Drawing for the job (mm, zero at the part's lowest x, y, z). Coordinates: 2 decimals unless noted, no trailing zeros. Loops run counter-clockwise (first coordinate to the right, second up) from the corner with the lowest first, then second, coordinate; pieces in that order, holes last. Notation, with made-up numbers: (-13, -24.75) - (27, -24.75) arc R3 ccw to (27, -20.75) - close; hole circle Ø11 at (-3.5, 2). An arc over 180 degrees is marked (long way). Put each result on its own line as item: value.
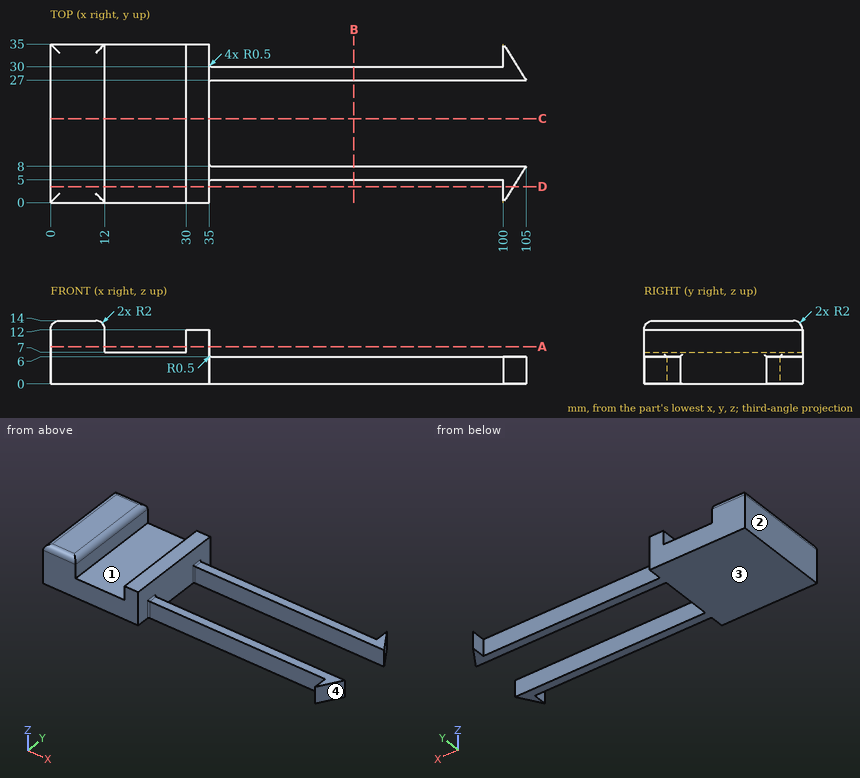
Q1. Pin check, flat tips, straight feed: pin 1 Ø4 at (x, y) = (81.5, 31.5) entering from +Z; pin 2 Ø3 at (x, z) = (78.5, 1.5) entering from +Y; pin 3 Ø3.5 at (y, z) = (10, 8.5) entering from +X. Stop position of each tip, or through.
Determined:
pin 1: z = 6
pin 2: y = 30
pin 3: x = 35
Q2. Mould opens along X. For the marked faces 1, 2, 3 and 4 say: +X half, -X half, draft (parallel to the pull), parting line (faces both ways), or undercut.
Determined:
face 1: undercut
face 2: -X half
face 3: draft
face 4: +X half
Q3. Slice it at D-D, the plane y = 3.5. Give the cut face in (x, z), then the cut area to 3 significant figures.
Determined:
outline: (0, 0) - (35, 0) - (35, 12) - (30, 12) - (30, 7) - (12, 7) - (12, 12) arc R2 ccw to (10, 14) - (2, 14) arc R2 ccw to (0, 12) - close; (100, 0) - (102.19, 0) - (102.19, 6) - (100, 6) - close
area: 365 mm2
Q4. Wall check: L1, parallel to X at y = 3.5, z = 11.25; L2, parallel to Y at x = 60.5, z = 4; L3, parallel to Z at x = 19.5, y = 5. Give the ranges that are in metal, low to high. Write a range as from..to.
Determined:
L1: 0..12, 30..35
L2: 5..8, 27..30
L3: 0..7
Q5. Slice it at A-A, the plane z = 8.25. Give the cut face in (x, y).
Determined:
outline: (0, 0) - (12, 0) - (12, 35) - (0, 35) - close; (30, 0) - (35, 0) - (35, 35) - (30, 35) - close
Q6. Slice it at B-B, the plane x = 67. Give the cut face in (y, z), then the cut area to 3 significant figures.
Determined:
outline: (5, 0) - (8, 0) - (8, 6) - (5, 6) - close; (27, 0) - (30, 0) - (30, 6) - (27, 6) - close
area: 36.0 mm2
Q7. Slice it at C-C, the plane y = 18.5. Give the cut face in (x, z).
Determined:
outline: (0, 0) - (35, 0) - (35, 12) - (30, 12) - (30, 7) - (12, 7) - (12, 12) arc R2 ccw to (10, 14) - (2, 14) arc R2 ccw to (0, 12) - close
